Build history of the part. All positions in model axes, mm. A direction names the side the tool comes from. Round coordinates to 2 decimals unless told otherwise and drop trailing zeros. Write each loop counter-clockwise with the first axis right and the second up, starting at its lowest first coordinate (ties: lowest second). Pieces come first, ordered by that corner, then holes.
Item 1: Drop flat-ended pins along their axis: pin 1 Ø5 at (y, z) = (-2, -28.5) entering from +X; pin 2 Ø8 at (x, z) = (-29.5, -15) entering from -Y; pin 3 Ø3 at (x, z) = (-115, -5) entering from -Y. Give the stop position or say it passes through.
Item 2: 3-axis set-ups, long thin cutter, end or side, ignore diameter. For faces 1 (the flat face through (-127, 0, -16)), 2 (the flat face through (-77, 1.778, -16)): which of +Z, -Z, +X, -X, +Y, -Y reach the whole face in a straight line?
Item 3: Band-saw the part on B-B, the plane z = -13. Write the cut outline in (x, y), then the cut area to 3 significant figures.
Item 4: Band-saw the part on D-D, the plane x = -140.5. Write the cut outline in (y, z).
Item 5: Band-saw the part on A-A, the plane x = -106. Write the cut outline in (y, z).
Item 6: Mould opens along Z. For faces 3 (the flat face through (0, -3, -16)), 4 (the flat face through (-77, -3, 0)), 5 (the flat face through (-112, 1.524, -26)) say: +Z half, -Z half, draft (parallel to the pull), parting line (faces both ways), or undercut.
Item 7: Band-saw the part on C-C, the plane y = -6. Write the cut outline in (x, z).
Item 8: Wall check: probe 1 along X at (y, z) = (-7.5, -21.5); probe 2 along Z at (x, y) = (-6.5, -2.5); probe 3 along X at (y, z) = (-1, -13.5). Give the ranges that are in metal, low to high.
Autodesk Inventor part; units mm, degrees
ref_plane "YZ Plane" through (0, 0, 0) normal (1, 0, 0) x (0, 1, 0)
ref_plane "XZ Plane" through (0, 0, 0) normal (0, 1, 0) x (-1, 0, 0)
ref_plane "XY Plane" through (0, 0, 0) normal (0, 0, 1) x (1, 0, 0)
sketch "Sketch1" plane through (0, 0, 0) normal (0, 1, 0) x (-1, 0, 0)
  line L0 (0, 0) -> (152.4, 0)
  line L1 (152.4, 0) -> (152.4, -31.75)
  line L2 (152.4, -31.75) -> (0, -31.75)
  line L3 (0, -31.75) -> (0, 0)
  line L4 (127, -8.89) -> (96.52, -8.89)
  line L5 (96.52, -8.89) -> (96.52, -22.86)
  line L6 (96.52, -22.86) -> (127, -22.86)
  line L7 (127, -22.86) -> (127, -8.89)
  line L8 (117.2368, -8.89) -> (117.2368, 0)
  line L9 (117.2368, -22.86) -> (117.2368, -31.75)
  dimension "d0" = 152.4
  dimension "d1" = 31.75
  dimension "d2" = 30.48
  dimension "d3" = 13.97
  dimension "d4" = 25.4
extrude "Extrusion1" add sketch "Sketch1" along normal blind 1.778 contours L0 L8 L4 L5 L6 L9 L2 L3 | L0 L1 L2 L9 L6 L7 L4 L8
sketch "Sketch2" plane through (0, 0, 0) normal (0, -1, 0) x (1, 0, 0)
  line L0 (-152.4, 0) -> (0, 0)
  line L1 (0, 0) -> (0, -31.75)
  line L2 (-152.4, 0) -> (0, 0)
  line L3 (0, 0) -> (0, -31.75)
  line L4 (0, -31.75) -> (-152.4, -31.75)
  line L5 (-152.4, -31.75) -> (-152.4, 0)
  line L6 (-127, -2.7348) -> (-96.52, -2.7348)
  line L7 (-96.52, -2.7348) -> (-96.52, -29.0152)
  line L8 (-96.52, -29.0152) -> (-127, -29.0152)
  line L9 (-127, -29.0152) -> (-127, -2.7348)
  line L10 (-127, -8.89) -> (-127, -22.86)
  line L11 (-103.8171, -2.7348) -> (-103.8171, 0)
  line L12 (-104.7941, -29.0152) -> (-104.7941, -31.75)
  line L13 (0, -31.75) -> (-152.4, -31.75)
  dimension "d7" = 30.48
  dimension "d8" = 0
extrude "Extrusion2" add sketch "Sketch2" along normal blind 1.778 contours L0 L11 L6 L9 L8 L12 L4 L5 | L0 L1 L4 L12 L8 L7 L6 L11
sketch "Sketch3" plane through (0, -1.778, 0) normal (0, -1, 0) x (1, 0, 0)
  line L0 (-152.4, 0) -> (0, 0)
  line L1 (0, -31.75) -> (-152.4, -31.75)
  line L2 (-152.4, 0) -> (0, 0)
  line L3 (0, 0) -> (0, -31.75)
  line L4 (0, -31.75) -> (-152.4, -31.75)
  line L5 (-152.4, -31.75) -> (-152.4, 0)
  line L6 (-1.5875, -30.1625) -> (-1.5875, -1.5875)
  line L7 (-1.5875, -1.5875) -> (-150.8125, -1.5875)
  line L8 (-150.8125, -1.5875) -> (-150.8125, -30.1625)
  line L9 (-150.8125, -30.1625) -> (-1.5875, -30.1625)
  dimension "d11" = 1.5875
extrude "Extrusion3" add sketch "Sketch3" along normal blind 6.35
sketch "Sketch4" plane through (0, 1.778, 0) normal (0, 1, 0) x (1, 0, 0)
  line L0 (-152.4, 0) -> (0, 0)
  line L1 (-152.4, 31.75) -> (-152.4, 0)
  line L2 (0, 0) -> (-152.4, 0)
  line L3 (-152.4, 0) -> (-152.4, 31.75)
  line L4 (-152.4, 31.75) -> (0, 31.75)
  line L5 (-6.35, 25.4) -> (-146.05, 25.4)
  line L6 (-146.05, 25.4) -> (-146.05, 6.35)
  line L7 (-146.05, 6.35) -> (-6.35, 6.35)
  line L8 (-13.5859, 25.4) -> (0, 25.4)
  line L9 (0, 0) -> (0, 31.75)
  line L10 (-13.5859, 6.35) -> (0, 6.35)
  line L11 (0, 31.75) -> (0, 25.4)
  line L12 (0, 6.35) -> (0, 0)
  line L13 (-127, 22.86) -> (-96.52, 22.86)
  line L14 (-96.52, 22.86) -> (-93.98, 22.86)
  line L15 (-93.98, 22.86) -> (-93.98, 25.4)
  line L16 (-93.98, 25.4) -> (-96.52, 25.4)
  line L17 (-96.52, 25.4) -> (-96.52, 22.86)
  line L18 (-96.52, 2.7348) -> (-96.52, 29.0152)
  line L19 (-96.52, 6.35) -> (-93.98, 6.35)
  line L20 (-93.98, 6.35) -> (-93.98, 8.89)
  line L21 (-93.98, 8.89) -> (-96.52, 8.89)
  line L22 (-96.52, 8.89) -> (-96.52, 6.35)
  line L23 (-121.92, 25.4) -> (-124.46, 25.4)
  line L24 (-124.46, 25.4) -> (-124.46, 22.86)
  line L25 (-124.46, 22.86) -> (-121.92, 22.86)
  line L26 (-121.92, 22.86) -> (-121.92, 25.4)
  line L27 (-121.92, 6.35) -> (-124.46, 6.35)
  line L28 (-124.46, 6.35) -> (-124.46, 8.89)
  line L29 (-124.46, 8.89) -> (-121.92, 8.89)
  line L30 (-121.92, 8.89) -> (-121.92, 6.35)
  line L31 (-68.58, 25.4) -> (-66.04, 25.4)
  line L32 (-66.04, 25.4) -> (-66.04, 22.86)
  line L33 (-66.04, 22.86) -> (-68.58, 22.86)
  line L34 (-68.58, 22.86) -> (-68.58, 25.4)
  line L35 (-68.58, 6.35) -> (-66.04, 6.35)
  line L36 (-66.04, 6.35) -> (-66.04, 8.89)
  line L37 (-66.04, 8.89) -> (-68.58, 8.89)
  line L38 (-68.58, 8.89) -> (-68.58, 6.35)
  line L39 (-40.64, 6.35) -> (-38.1, 6.35)
  line L40 (-38.1, 6.35) -> (-38.1, 8.89)
  line L41 (-38.1, 8.89) -> (-40.64, 8.89)
  line L42 (-40.64, 8.89) -> (-40.64, 6.35)
  line L43 (-40.64, 25.4) -> (-38.1, 25.4)
  line L44 (-38.1, 25.4) -> (-38.1, 22.86)
  line L45 (-38.1, 22.86) -> (-40.64, 22.86)
  line L46 (-40.64, 22.86) -> (-40.64, 25.4)
  line L47 (-12.7, 25.4) -> (-10.16, 25.4)
  line L48 (-10.16, 25.4) -> (-10.16, 22.86)
  line L49 (-10.16, 22.86) -> (-12.7, 22.86)
  line L50 (-12.7, 22.86) -> (-12.7, 25.4)
  line L51 (-12.7, 6.35) -> (-10.16, 6.35)
  line L52 (-10.16, 6.35) -> (-10.16, 8.89)
  line L53 (-10.16, 8.89) -> (-12.7, 8.89)
  line L54 (-12.7, 8.89) -> (-12.7, 6.35)
  point P0 (-121.92, 7.62)
  point P1 (-96.52, 7.62)
  point P2 (-93.98, 24.13)
  point P3 (-68.58, 24.13)
  point P4 (-40.64, 24.13)
  point P5 (-66.04, 24.13)
  point P6 (-12.7, 24.13)
  point P7 (-38.1, 24.13)
  point P8 (-6.35, 6.35)
  dimension "d14" = 6.35
  dimension "d15" = 2.54
  dimension "d16" = 2.54
  dimension "d17" = 2.54
  dimension "d18" = 2.54
  dimension "d19" = 2.54
  dimension "d20" = 2.54
  dimension "d21" = 25.4
  dimension "d22" = 2.54
  dimension "d23" = 2.54
  dimension "d24" = 2.54
  dimension "d25" = 2.54
  dimension "d26" = 2.54
  dimension "d27" = 2.54
  dimension "d28" = 2.54
  dimension "d29" = 2.54
  dimension "d30" = 2.54
  dimension "d31" = 2.54
  dimension "d32" = 2.54
  dimension "d33" = 2.54
  dimension "d34" = 25.4
  dimension "d35" = 25.4
  dimension "d36" = 25.4
extrude "Extrusion4" add sketch "Sketch4" along normal blind 31.75 contours L1 L4 L9 L8 L5 L6 L7 L10 L0 | L7 L54 L53 L52 | L48 L49 L50 L5 | L7 L42 L41 L40 | L44 L45 L46 L5 | L7 L38 L37 L36 | L32 L33 L34 L5 | L7 L18 L21 L20 | L15 L14 L17 L5 | L7 L28 L29 L30 | L26 L13 L24 L5
sketch "Sketch5" plane through (-93.98, 1.778, -8.89) normal (0, 0, -1) x (-1, 0, 0)
  line L0 (2.54, 31.75) -> (0, 31.75)
  line L1 (0, 31.75) -> (0, 29.21)
  line L2 (0, 29.21) -> (2.54, 29.21)
  line L3 (2.54, 29.21) -> (2.54, 31.75)
  line L4 (30.48, 31.75) -> (27.94, 31.75)
  line L5 (30.48, 0) -> (30.48, 31.75)
  line L6 (27.94, 31.75) -> (30.48, 31.75)
  line L7 (30.48, 31.75) -> (30.48, 29.21)
  line L8 (30.48, 29.21) -> (27.94, 29.21)
  line L9 (27.94, 29.21) -> (27.94, 31.75)
  line L10 (-27.94, 0) -> (-27.94, 31.75)
  line L11 (-25.4, 0) -> (-25.4, 31.75)
  line L12 (-27.94, 29.21) -> (-25.4, 29.21)
  line L13 (-25.4, 29.21) -> (-25.4, 31.75)
  line L14 (-25.4, 31.75) -> (-27.94, 31.75)
  line L15 (-27.94, 31.75) -> (-27.94, 29.21)
  line L16 (-93.98, 31.75) -> (58.42, 31.75)
  line L17 (-27.94, 31.75) -> (-25.4, 31.75)
  line L18 (-25.4, 31.75) -> (-25.4, 29.21)
  line L19 (-25.4, 29.21) -> (-27.94, 29.21)
  line L20 (-27.94, 29.21) -> (-27.94, 31.75)
  line L21 (-53.34, 31.75) -> (-55.88, 31.75)
  line L22 (-55.88, 31.75) -> (-55.88, 29.21)
  line L23 (-55.88, 29.21) -> (-53.34, 29.21)
  line L24 (-53.34, 29.21) -> (-53.34, 31.75)
  line L25 (-81.28, 31.75) -> (-83.82, 31.75)
  line L26 (-83.82, 31.75) -> (-83.82, 29.21)
  line L27 (-83.82, 29.21) -> (-81.28, 29.21)
  line L28 (-81.28, 29.21) -> (-81.28, 31.75)
  line L29 (30.48, 31.75) -> (52.07, 31.75)
  line L30 (30.48, 31.75) -> (27.94, 31.75)
  line L31 (27.94, 31.75) -> (27.94, 29.21)
  line L32 (27.94, 29.21) -> (30.48, 29.21)
  line L33 (30.48, 29.21) -> (30.48, 31.75)
  point P0 (-93.98, -1.778)
  point P1 (0, 30.48)
  point P2 (-25.4, 30.48)
  point P3 (-27.94, 30.48)
  point P4 (-53.34, 30.48)
  point P5 (-81.28, 30.48)
  point P6 (-55.88, 30.48)
  point P7 (27.94, 30.48)
  point P8 (2.54, 30.48)
  dimension "d39" = 2.54
  dimension "d40" = 2.54
  dimension "d41" = 2.54
  dimension "d42" = 2.54
  dimension "d43" = 2.54
  dimension "d44" = 2.54
  dimension "d45" = 25.4
  dimension "d46" = 25.4
  dimension "d47" = 2.54
  dimension "d48" = 2.54
  dimension "d49" = 25.4
  dimension "d50" = 2.54
  dimension "d51" = 2.54
  dimension "d52" = 25.4
extrude "Extrusion5" add sketch "Sketch5" along normal up to next
sketch "Sketch6" plane through (0, 33.528, 0) normal (0, 1, 0) x (1, 0, 0)
  line L0 (-152.4, 31.75) -> (-152.4, 0)
  line L1 (0, 31.75) -> (-152.4, 31.75)
  line L2 (-152.4, 0) -> (0, 0)
  line L3 (0, 0) -> (0, 31.75)
  line L4 (0, 31.75) -> (-152.4, 31.75)
  line L5 (-152.4, 31.75) -> (-152.4, 0)
extrude "Extrusion6" add sketch "Sketch6" along normal blind 3.175
ref_plane "Work Plane1" through (-127, 1.778, -8.89) normal (0.7071, -0.7071, 0) x (0, 0, -1)
sketch "Sketch7" plane through (-127, 1.778, -8.89) normal (0.7071, -0.7071, 0) x (0, 0, -1)
  line L0 (20.1252, -1.2572) -> (20.1252, 20.2954)
  line L1 (20.1252, 0) -> (-6.1552, 0)
  line L2 (-6.1552, 0) -> (-6.1552, 127)
  line L3 (-6.1552, 127) -> (20.1252, 127)
  line L4 (20.1252, 127) -> (20.1252, 0)
  line L5 (0, 0) -> (13.97, 0)
  point P0 (-8.89, 88.5453)
  point P1 (20.1252, 20.2954)
  dimension "d58" = 0
  dimension "d59" = 127
extrude "Extrusion7" cut sketch "Sketch7" against normal blind 3.175
sketch "Sketch8" plane through (0, 1.778, 0) normal (0, 1, 0) x (1, 0, 0)
  line L0 (63.8737, 171.7375) -> (-193.0507, 171.7375)
  line L1 (-193.0507, 171.7375) -> (-193.0507, -76.4775)
  line L2 (-193.0507, -76.4775) -> (63.8737, -76.4775)
  line L3 (63.8737, -76.4775) -> (63.8737, 171.7375)
  point P0 (0, 0)
extrude "Extrusion8" cut sketch "Sketch8" along normal up to next
sketch "Sketch9" plane through (0, 0, 0) normal (0, -1, 0) x (1, 0, 0)
  line L0 (-96.52, -2.7348) -> (-96.52, -29.0152)
  line L1 (-127, -29.0152) -> (-127, -2.7348)
  line L2 (-96.52, -3.6571) -> (-127, -3.6571)
  line L3 (-127, -3.6571) -> (-127, -7.587)
  line L4 (-127, -7.587) -> (-96.52, -7.587)
  line L5 (-96.52, -7.587) -> (-96.52, -3.6571)
  line L6 (-96.52, -24.0081) -> (-127, -24.0081)
  line L7 (-127, -24.0081) -> (-127, -28.0783)
  line L8 (-127, -28.0783) -> (-96.52, -28.0783)
  line L9 (-96.52, -28.0783) -> (-96.52, -24.0081)
  point P0 (0, 0)
extrude "Extrusion9" cut sketch "Sketch9" against normal blind 1.524 contours L0 L4 L1 L2 | L0 L8 L1 L6
properties part number "Base"
Results:
1. pin 1: stops at x = 0
1. pin 2: stops at y = -1.78
1. pin 3: stops at y = 0
2. face 1: -Y
2. face 2: +Z, -Z, +X, -X, +Y
3. outline: (-152.4, -8.13) - (-150.81, -8.13) - (-150.81, -1.78) - (-127, -1.78) - (-127, 1.78) - (-152.4, 1.78) - close; (-96.52, -1.78) - (-1.59, -1.78) - (-1.59, -8.13) - (0, -8.13) - (0, 1.78) - (-96.52, 1.78) - close
3. area: 454 mm2
4. outline: (-8.13, -31.75) - (1.78, -31.75) - (1.78, 0) - (-8.13, 0) - (-8.13, -1.59) - (-1.78, -1.59) - (-1.78, -30.16) - (-8.13, -30.16) - close
5. outline: (-8.13, -31.75) - (1.78, -31.75) - (1.78, -22.86) - (0, -22.86) - (0, -24.01) - (1.52, -24.01) - (1.52, -28.08) - (0, -28.08) - (0, -29.02) - (-1.78, -29.02) - (-1.78, -30.16) - (-8.13, -30.16) - close; (-8.13, -1.59) - (-1.78, -1.59) - (-1.78, -2.73) - (0, -2.73) - (0, -3.66) - (1.52, -3.66) - (1.52, -7.59) - (0, -7.59) - (0, -8.89) - (1.78, -8.89) - (1.78, 0) - (-8.13, 0) - close
6. face 3: draft
6. face 4: +Z half
6. face 5: undercut
7. outline: (-152.4, -31.75) - (0, -31.75) - (0, 0) - (-152.4, 0) - close; hole (-150.81, -30.16) - (-1.59, -30.16) - (-1.59, -1.59) - (-150.81, -1.59) - close
8. probe 1: x = -152.4 to -150.81, -1.59 to 0
8. probe 2: z = -31.75 to -30.16, -1.59 to 0
8. probe 3: x = -152.4 to -127, -96.52 to 0
